from build123d import *

# Parameters (mm, degrees)
FASE1_SIZE                      = 1
SKIZZE2_W                       = 3.5
SKIZZE2_H                       = 18
SCHNITT_LINEAR_AUSTRAGEN1_DEPTH = 10
SKIZZE3_R                       = 7.5
AUFSATZ_LINEAR_AUSTRAGEN1_DEPTH = 2


with BuildPart() as part:
    # Skizze1 → Rotation1 (revolve)
    with BuildSketch(Plane.XY):
        with BuildLine():
            Line((0, 0), (-55, 0))
            Line((-55, 0), (-55, 2))
            Line((-55, 2), (-60, 2))
            Line((-60, 2), (-60, 6.107169523))
            ThreePointArc((-60, 6.107169523), (-59.298133329, 8.035532352), (-57.520944533, 9.061592782))
            Line((-57.520944533, 9.061592782), (-12.5, 17))
            Line((-12.5, 17), (-12.5, 20))
            Line((-12.5, 20), (-10, 20))
            Line((-10, 20), (-10, 270))
            Line((-10, 270), (0, 270))
            Line((0, 270), (0, 0))
        make_face()
    revolve(axis=Axis((0, 290, 0), (0, -1, 0)))

    # Fase1
    fase1_edges = [part.edges().sort_by_distance(p)[0] for p in [
        (10, 270, 0),
    ]]
    chamfer(fase1_edges, length=FASE1_SIZE)

    # Skizze2 → Schnitt-Linear austragen1 (cut, symmetric)
    with BuildSketch(Plane.XY):
        with Locations((-8.25, 29)):
            Rectangle(SKIZZE2_W, SKIZZE2_H)
        with Locations((8.25, 29)):
            Rectangle(SKIZZE2_W, SKIZZE2_H)
    extrude(amount=SCHNITT_LINEAR_AUSTRAGEN1_DEPTH, both=True, mode=Mode.SUBTRACT)

    # Skizze3 → Aufsatz-Linear austragen1 (add)
    with BuildSketch(Plane.XZ.offset(-2)):
        with BuildLine():
            Line((0, 15), (0, -15))
            Line((0, -15), (80, -15))
            ThreePointArc((80, -15), (95, 0), (80, 15))
            Line((80, 15), (0, 15))
        make_face()
        with Locations((80, 0)):
            Circle(SKIZZE3_R, mode=Mode.SUBTRACT)
    extrude(amount=-AUFSATZ_LINEAR_AUSTRAGEN1_DEPTH)


solid = part.part
Here's how the part is built. I have some questions about the finished solid (model axes, mm). A direction names the side the tool comes from. Round coordinates to 2 decimals unless told otherwise and drop trailing zeros. Loops run counter-clockwise (first coordinate to the right, second up) from the corner with the lowest first, then second, coordinate; pieces in that order, holes last. Notation, with made-up numbers: (59.5, -39) - (65.5, -39) arc R10 cw to (65.5, -31) - close; hole circle Ø1 at (83.25, 72). An arc over 180 degrees is marked (long way). One line per question, with ' | ' between items. Start each with the question number.
Q1. I want a section at B-B (x = 0). Write out the boundary of the cut face in (y, z).
Q2. Will these pins go through, and if not, where does the flat tip stop? pin 1 (0.6 mm diameter, centred on x = 70.5, y = 3.5, fed in from +Z); pin 2 (24 mm diameter, centred on x = 80, z = 0, fed in from +Y); pin 3 (4.5 mm diameter, centred on y = 26.5, z = -3, fed in from +X).
Q3. For faces 1 (the flat face through (6.5, 29, 0)), 2 (the cylindrical face through (-9.54, 146.24, -3)), 3 (the cylindrical face through (11.923, 1.014, 53.692)), 4 (the flat face through (-8, 20, 0)), which set-ups out of +Z, -Z, +X, -X, +Y, -Y let a thin tool reach every point of the face, with its end or its side?
Q4. We'd pull the mould along Y, two halves only. Please class faces 5 (the cylindrical face through (95, 3, 0)), 6 (the flat face through (-6.5, 29, 0)), 7 (the flat face through (0, 270, 0)), 8 (the flat face through (52, 2, 22)): +Y half, -Y half, draft (parallel to the pull), parting line (faces both ways), or undercut.
Q5. I want a section at C-C (y = 143). Write out the boundary of the cut face in (x, z).
Q6. Please list where these lines run through material, in increasing order: line 1 (Z direction, x = 80, y = 2.8); line 2 (Y direction, x = 87, z = 6.5); line 3 (Y direction, x = 49, z = -4.5). Write a range as [from, to].
Q7. I want a section at D-D (x = 65). Write out the boundary of the cut face in (y, z), then the cut area to 3 significant figures.
Response values:
1) outline: (0, -55) - (2, -55) - (2, -60) - (6.11, -60) arc R3 ccw to (9.06, -57.52) - (17, -12.5) - (20, -12.5) - (20, -10) - (269, -10) - (270, -9) - (270, 9) - (269, 10) - (20, 10) - (20, 12.5) - (17, 12.5) - (9.06, 57.52) arc R3 ccw to (6.11, 60) - (2, 60) - (2, 55) - (0, 55) - close
2) pin 1: stops at z = 15 | pin 2: stops at y = 4 | pin 3: stops at x = 6.5
3) face 1: +Z, -Z, +X | face 2: +Y | face 3: -Y | face 4: none
4) face 5: draft | face 6: undercut | face 7: +Y half | face 8: -Y half
5) outline: circle Ø20 at (0, 0)
6) line 1: z = [-15, -7.5], [7.5, 15] | line 2: y = [2, 4] | line 3: y = [0, 10.53]
7) outline: (2, -15) - (4, -15) - (4, 15) - (2, 15) - close | area: 60.0 mm²
